Check sheet for the drawn part. Datum: minimum x, y, z corner. Units: mm. Coordinates: 2 decimals unless noted, no trailing zeros. Loops run counter-clockwise (first coordinate to the right, second up) from the corner with the lowest first, then second, coordinate; pieces in that order, holes last. Notation, with made-up numbers: M 18.25,-30.75 L 38.25,-30.75 A29 ccw 38.25,4.25 Z; hole C 22,8.25 d2. An arc over 180 degrees is marked long. Use CSV: the item, a comma, the result in double quotes. Start each with the question number.
(1) Section check A-A on y = 35. Record the cut outline in (x, z), and give its area (3 significant figures).
(2) Section check B-B on z = 25. Record the cut outline in (x, y), and give its area (3 significant figures).
(3) Scan lines: line 1 (Y direction, x = 2.2, z = 25); line 2 (Z direction, x = 1.3, y = 31); line 3 (Z direction, x = 1.35, y = 65). Record each from-to range of solid material in increasing order.
(4) Go/stop test with flat-tipped pins: pin 1 Ø1 at (y, z) = (59.5, 11) entering from +X; pin 2 Ø1 at (x, z) = (1.5, 39.5) entering from +Y; pin 3 Ø1.5 at (x, z) = (0.5, 41) entering from +Y; pin 4 Ø1 at (x, z) = (0.5, 36.5) entering from -Y. Record where each tip stops, or that it passes through.
(5) Section check D-D on y = 24. Record the cut outline in (x, z).
(6) Section check C-C on x = 0.8. Record the cut outline in (y, z), and give its area (3 significant figures).
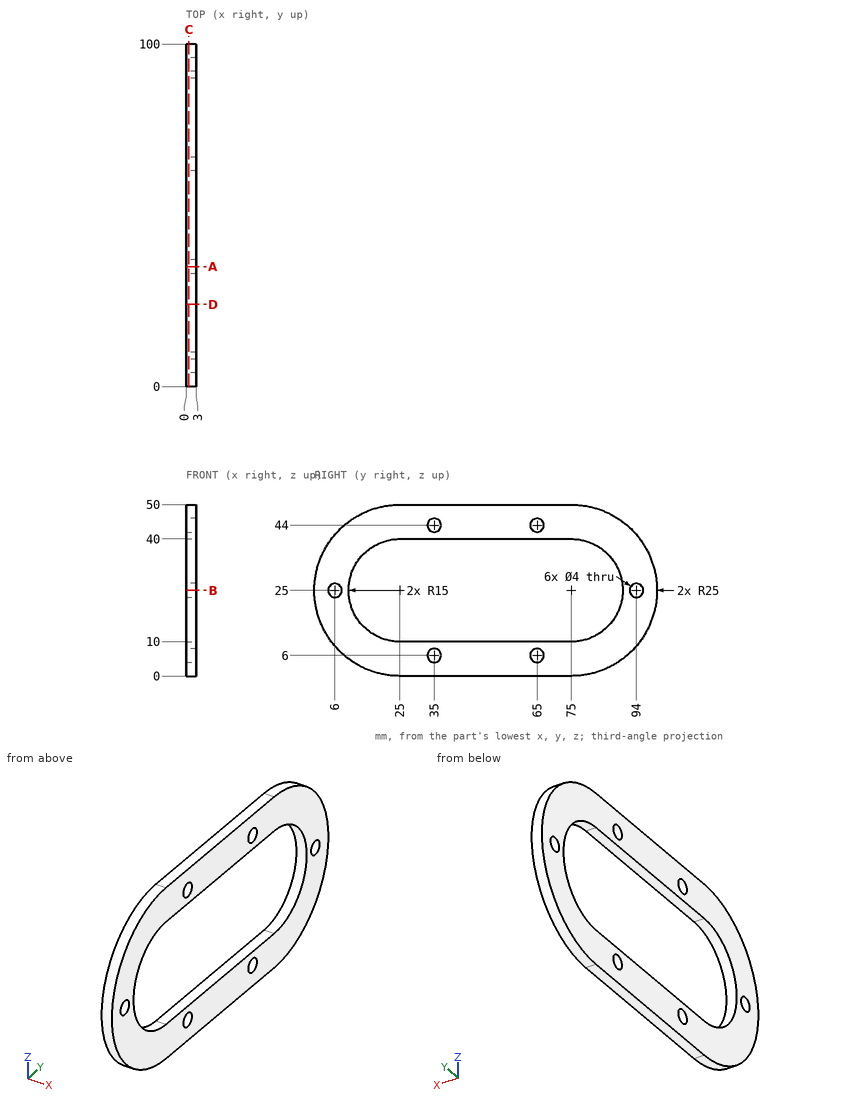
Outcome:
1,outline,"M 0,0 L 3,0 L 3,4 L 0,4 Z; M 0,8 L 3,8 L 3,10 L 0,10 Z; M 0,40 L 3,40 L 3,42 L 0,42 Z; M 0,46 L 3,46 L 3,50 L 0,50 Z"
1,area,"36.0 mm²"
2,outline,"M 0,0 L 3,0 L 3,4 L 0,4 Z; M 0,8 L 3,8 L 3,10 L 0,10 Z; M 0,90 L 3,90 L 3,92 L 0,92 Z; M 0,96 L 3,96 L 3,100 L 0,100 Z"
2,area,"36.0 mm²"
3,line 1,"y = 0 to 4, 8 to 10, 90 to 92, 96 to 100"
3,line 2,"z = 0 to 10, 40 to 50"
3,line 3,"z = 0 to 4, 8 to 10, 40 to 42, 46 to 50"
4,pin 1,"passes through"
4,pin 2,"stops at y = 95.71"
4,pin 3,"stops at y = 94.81"
4,pin 4,"stops at y = 2.55"
5,outline,"M 0,0.02 L 3,0.02 L 3,10.03 L 0,10.03 Z; M 0,39.97 L 3,39.97 L 3,49.98 L 0,49.98 Z"
6,outline,"M 25,0 L 75,0 A25 ccw 75,50 L 25,50 A25 ccw Z; hole C 6,25 d4; hole M 25,10 L 75,10 A15 ccw 75,40 L 25,40 A15 ccw Z; hole C 35,6 d4; hole C 35,44 d4; hole C 65,6 d4; hole C 65,44 d4; hole C 94,25 d4"
6,area,"2,180 mm²"
